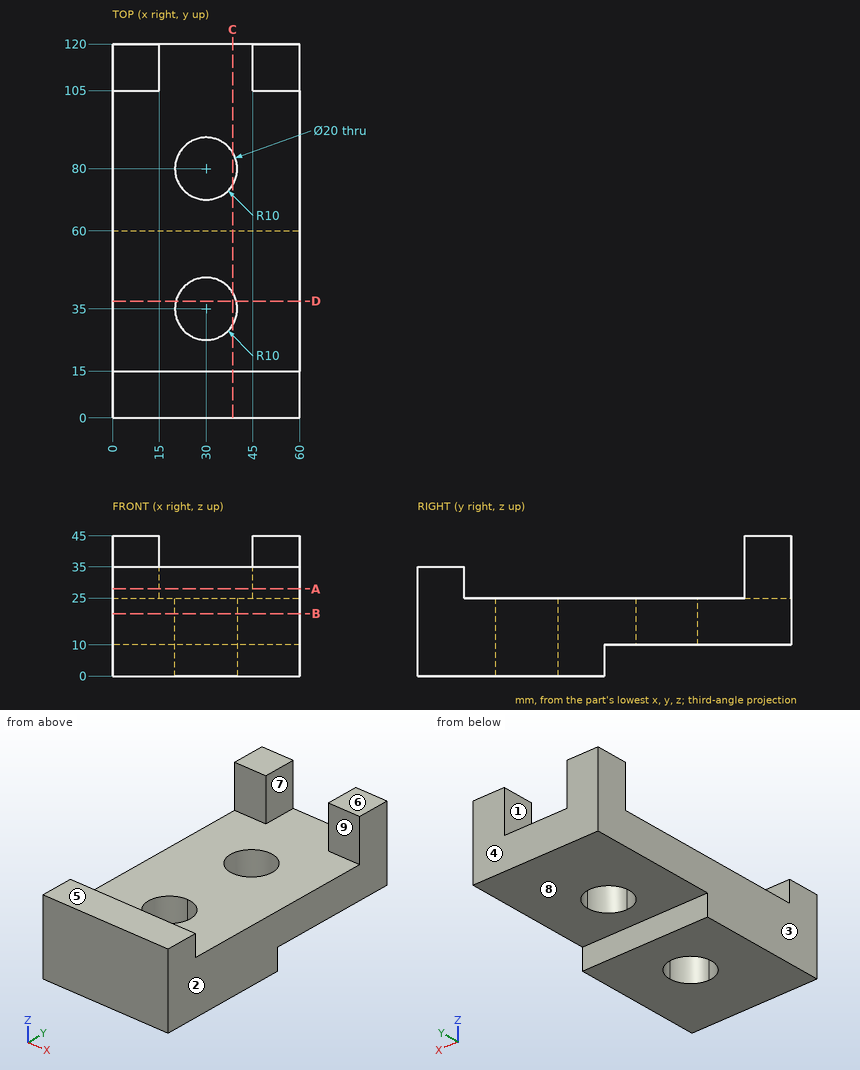
Job drawing, mm, ordinate dimensions from the low corner. One solid piece. A direction names the side the tool comes from. Coordinates: 2 decimals unless noted, no trailing zeros. Order: outer loops, then holes, each group sorted by start corner. A loop starts at its lowest first (then second) coordinate and runs counter-clockwise, first axis right, second up. Notation, with made-up numbers: M 65,63.5 L 121,63.5 A10 ccw 121,76.5 Z; hole C 43.5,4.25 d8. An arc over 180 degrees is marked long. Return JSON: item names as keys, results as strings.
1. Saw through at A-A (z = 28). Give the cut face in (x, y).
Ans:
{"outline": "M 0,0 L 60,0 L 60,15 L 0,15 Z; M 0,105 L 15,105 L 15,120 L 0,120 Z; M 45,105 L 60,105 L 60,120 L 45,120 Z"}
2. Saw through at D-D (y = 37.5). Give the cut face in (x, z).
Ans:
{"outline": "M 0,0 L 20.32,0 L 20.32,25 L 0,25 Z; M 39.68,0 L 60,0 L 60,25 L 39.68,25 Z"}
3. Saw through at C-C (x = 38.5). Give the cut face in (y, z), and give its area (3 significant figures).
Ans:
{"outline": "M 0,0 L 29.73,0 L 29.73,25 L 15,25 L 15,35 L 0,35 Z; M 40.27,0 L 60,0 L 60,10 L 74.73,10 L 74.73,25 L 40.27,25 Z; M 85.27,10 L 120,10 L 120,25 L 85.27,25 Z", "area": "2,130 mm^2"}
4. Tool access for the marked faces 5, 6, 7, 8 and 9: list every direction of +Z, -Z, +X, -X, +Y, -Y with a clear straight run to the whole face (end or side of a thin tool).
Ans:
{"face 5": "+Z, +X, -X, -Y", "face 6": "+Z, +X, -X, +Y, -Y", "face 7": "+Z, +Y", "face 8": "-Z, +X, -X, +Y", "face 9": "+Z, +X, -X"}
5. Pull direction X, two halves, no side cores. Call the marked faces 1, 2, 3 and 4: +X half, -X half, draft (parallel to the pull), parting line (faces both ways), or undercut.
Ans:
{"face 1": "undercut", "face 2": "+X half", "face 3": "-X half", "face 4": "draft"}
6. Drill centre lines: probe 1 along Y at (x, z) = (30, 15); probe 2 along X at (y, z) = (80, 15); probe 3 along Y at (x, z) = (47, 29.5). Where is each one in solid material? Low to high.
Ans:
{"probe 1": "0 to 25, 45 to 70, 90 to 120", "probe 2": "0 to 20, 40 to 60", "probe 3": "0 to 15, 105 to 120"}
7. Saw through at B-B (z = 20). Give the cut face in (x, y).
Ans:
{"outline": "M 0,0 L 60,0 L 60,120 L 0,120 Z; hole C 30,80 d20; hole M 30,45 A10 ccw long 40,35 A10 ccw Z"}
8. Flat gauge pins, fed straight in: pin 1 (12 mm diameter, centred on y = 89.5, z = 36, fed in from -X); pin 2 (3 mm diameter, centred on x = 35.5, z = 4.5, fed in from +Y); pin 3 (6 mm diameter, centred on x = 45.5, y = 68, fed in from +Z); pin 4 (4.5 mm diameter, centred on x = 31, y = 10, fed in from +Z). Where does each tip first touch, or does it go through?
Ans:
{"pin 1": "through", "pin 2": "y = 60", "pin 3": "z = 25", "pin 4": "z = 35"}
